Geometry: final body of the model. Coordinates: model frame, mm. Face numbers are marked on the shaded views. A direction names the side the tool comes from. Coordinates: 2 decimals unless noted, no trailing zeros. Order: outer loops, then holes, each group sorted by start corner. A loop starts at its lowest first (then second) coordinate and runs counter-clockwise, first axis right, second up. Notation, with made-up numbers: M 62.25,38.5 L 82.25,38.5 A8 ccw 82.25,44.5 Z; hole C -32,20.5 d6. An arc over 180 degrees is marked long. Write item = value, one per line.
from build123d import *

# Parameters (mm, degrees)
SKETCH1_W               = 38.1
SKETCH1_H               = 38.1
BOSS_EXTRUDE1_DEPTH     = 4.572
SKETCH5_W               = 27.178
SKETCH5_H               = 27.178
BOSS_EXTRUDE2_DEPTH     = 19.812
SKETCH2_R               = 7.06349997
CUT_EXTRUDE1_DEPTH      = 20.812
F_1_4_20_TAPPED_HOLE1_D = 6.35
SKETCH6_W               = 11.986676998
SKETCH6_H               = 38.1
BOSS_EXTRUDE3_DEPTH     = 4.826


with BuildPart() as part:
    # Sketch1 → Boss-Extrude1 (new body)
    with BuildSketch(Plane(origin=(0, 0, 0), x_dir=(1, 0, 0), z_dir=(0, 1, 0))):
        Rectangle(SKETCH1_W, SKETCH1_H)
    extrude(amount=BOSS_EXTRUDE1_DEPTH)

    # Sketch5 → Boss-Extrude2 (add)
    with BuildSketch(Plane(origin=(0, 0, 0), x_dir=(1, 0, 0), z_dir=(0, 1, 0))):
        Rectangle(SKETCH5_W, SKETCH5_H)
    extrude(amount=BOSS_EXTRUDE2_DEPTH)

    # Sketch2 → Cut-Extrude1 (cut, through all)
    with BuildSketch(Plane.XZ):
        with Locations((0, 19)):
            Circle(SKETCH2_R)
    extrude(amount=-CUT_EXTRUDE1_DEPTH, mode=Mode.SUBTRACT)

    # 1/4-20 Tapped Hole1 (through all)
    with Locations(Plane(origin=(0, 0, 0), x_dir=(-1, 0, 0), z_dir=(0, -1, 0))):
        with Locations((0, 0)):
            Hole(F_1_4_20_TAPPED_HOLE1_D / 2)

    # Sketch6 → Boss-Extrude3 (add)
    with BuildSketch(Plane.XZ):
        with Locations((13.056661501, 0)):
            Rectangle(SKETCH6_W, SKETCH6_H)
        with Locations((-13.056661501, 0)):
            Rectangle(SKETCH6_W, SKETCH6_H)
    extrude(amount=BOSS_EXTRUDE3_DEPTH)


solid = part.part
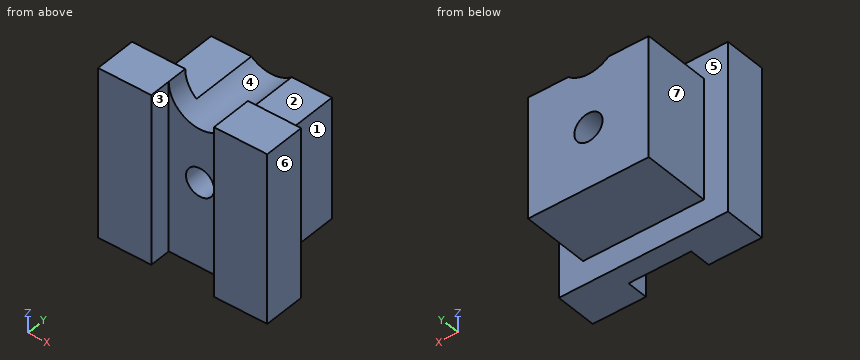
1) Mould query, pull axis X, two halves, no side actions, for the marked faces 4, 5, 6 and 7. Classes: pulls with the +X half, pulls with the -X half, needs draft (parallel to the pull), parting line crosses it, or undercut.
Numbers:
face_4 = undercut
face_5 = needs draft
face_6 = pulls with the +X half
face_7 = pulls with the -X half
2) Pin query (flat end, axial travel): pin 1 (6 mm diameter, centred on x = 4, y = 10.5, fed in from -Z); pin 2 (7 mm diameter, centred on x = -8, y = 12, fed in from +Z); pin 3 (12 mm diameter, centred on y = 14.5, z = -3, fed in from -X). Return the tip coordinate at first contact, or that it passes through.
Numbers:
pin_1 = -13.59
pin_2 = 13.59
pin_3 = -13.59
3) Line query: L1, parallel to Z at x = 0, y = 15 (1 decimal); L2, parallel to Z at x = 12, y = 17.75. Output: solid intervals per line, ascending.
Numbers:
L1 = -13.6 to -3.2, 3.2 to 11.9
L2 = -13.59 to 13.59
4) Set-up query: the marked faces 1, 2 and 3. Return all of +Z, -Z, +X, -X, +Y, -Y with unobstructed straight access to the full face (end or side cutting, diameter ignored); none if empty.
Numbers:
face_1 = +Z, -Z, +X, +Y
face_2 = +Z, +X, -X, +Y
face_3 = +Z, -Z, -Y
5) Section D-D, the plane x = 11. Return loops of the section in (y, z).
Numbers:
outline = M -4.83,-19.05 L 4.57,-19.05 L 4.57,-13.59 L 19.81,-13.59 L 19.81,13.59 L 4.57,13.59 L 4.57,19.05 L -4.83,19.05 Z
6) Section A-A, the plane z = 0. Return loops of the section in (x, y) (3 decimals).
Numbers:
outline = M -19.05,-4.826 L -7.063,-4.826 L -7.063,0 L -3.175,0 L -3.175,19.812 L -13.589,19.812 L -13.589,4.572 L -19.05,4.572 Z; M 3.175,0 L 7.063,0 L 7.063,-4.826 L 19.05,-4.826 L 19.05,4.572 L 13.589,4.572 L 13.589,19.812 L 3.175,19.812 Z
